Read the model definition and answer for the solid it produces. Units are mm, in the model's axes. A direction names the side the tool comes from. Coordinates: 2 decimals unless noted, no trailing zeros. Write each loop counter-clockwise with the first axis right and the second up, starting at its lowest first coordinate (ties: lowest second). Pieces come first, ordered by that corner, then holes. Notation, with made-up numbers: (-24.75, -30.75) -> (31.25, -30.75) arc R15 ccw to (31.25, -8.75) -> close; hole circle Ø2 at (-31, -37.75). An arc over 180 degrees is marked (long way). Return JSON: item names as keys, results as strings.
from build123d import *

# Parameters (mm, degrees)
SKETCH1_W           = 14.605
SKETCH1_H           = 46.482
SKETCH1_R           = 1.905
BOSS_EXTRUDE1_DEPTH = 44.45
SKETCH2_W           = 4.445
SKETCH2_H           = 33.02
CUT_EXTRUDE1_DEPTH  = 38.1
SKETCH3_W           = 42.545
SKETCH3_H           = 25.4
CUT_EXTRUDE2_DEPTH  = 12.065
CUT_EXTRUDE3_DEPTH  = 40.64
SKETCH5_W           = 25.4
SKETCH5_H           = 46.482
BOSS_EXTRUDE2_DEPTH = 3.81
FILLET1_R           = 2.54
FILLET2_R           = 1.016
CHAMFER1_SIZE       = 7.62
BOSS_EXTRUDE3_START = -7.62
BOSS_EXTRUDE3_DEPTH = 2.54
FILLET4_R           = 2.54


with BuildPart() as part:
    # Sketch1 → Boss-Extrude1 (new body)
    with BuildSketch(Plane.XY):
        with Locations((7.3025, 23.241)):
            Rectangle(SKETCH1_W, SKETCH1_H)
        with Locations((4.191, 42.291)):
            Circle(SKETCH1_R, mode=Mode.SUBTRACT)
        with Locations((4.191, 4.191)):
            Circle(SKETCH1_R, mode=Mode.SUBTRACT)
    extrude(amount=BOSS_EXTRUDE1_DEPTH)

    # Sketch2 → Cut-Extrude1 (cut)
    with BuildSketch(Plane.XY.offset(44.45)):
        with Locations((11.1125, 23.241)):
            Rectangle(SKETCH2_W, SKETCH2_H)
    extrude(amount=-CUT_EXTRUDE1_DEPTH, mode=Mode.SUBTRACT)

    # Sketch3 → Cut-Extrude2 (cut)
    with BuildSketch(Plane.ZY.offset(-13.335)):
        with Locations((21.2725, 23.241)):
            Rectangle(SKETCH3_W, SKETCH3_H)
    extrude(amount=CUT_EXTRUDE2_DEPTH, mode=Mode.SUBTRACT)

    # Sketch4 → Cut-Extrude3 (cut)
    with BuildSketch(Plane.XY.offset(44.45)):
        with BuildLine():
            Line((4.191, 38.1), (0, 38.1))
            Line((0, 38.1), (0, 46.482))
            Line((0, 46.482), (8.382, 46.482))
            Line((8.382, 46.482), (8.382, 42.291))
            ThreePointArc((8.382, 42.291), (7.15448452, 39.32751548), (4.191, 38.1))
        make_face()
        with BuildLine():
            Line((4.191, 8.382), (0, 8.382))
            Line((0, 8.382), (0, 0))
            Line((0, 0), (8.382, 0))
            Line((8.382, 0), (8.382, 4.191))
            ThreePointArc((8.382, 4.191), (7.15448452, 7.15448452), (4.191, 8.382))
        make_face()
    extrude(amount=-CUT_EXTRUDE3_DEPTH, mode=Mode.SUBTRACT)

    # Sketch5 → Boss-Extrude2 (add)
    with BuildSketch(Plane(origin=(0, 0, 0), x_dir=(-1, 0, 0), z_dir=(0, 0, -1))):
        with Locations((-27.305, 23.241)):
            Rectangle(SKETCH5_W, SKETCH5_H)
    extrude(amount=-BOSS_EXTRUDE2_DEPTH)

    # Fillet1
    fillet1_edges = [part.edges().sort_by_distance(p)[0] for p in [
        (8.382, 46.482, 24.13),
        (0, 38.1, 24.13),
        (0, 8.382, 24.13),
        (8.382, 0, 24.13),
        (0, 0, 1.905),
        (14.605, 0, 24.13),
        (14.605, 46.482, 24.13),
        (0, 46.482, 1.905),
        (40.005, 0, 1.905),
        (40.005, 46.482, 1.905),
    ]]
    fillet(fillet1_edges, radius=FILLET1_R)

    # Fillet2
    fillet2_edges = [part.edges().sort_by_distance(p)[0] for p in [
        (11.4935, 0, 44.45),
        (0, 23.241, 44.45),
        (11.4935, 46.482, 44.45),
        (8.382, 3.3655, 44.45),
        (14.605, 23.241, 44.45),
        (3.3655, 38.1, 44.45),
        (13.861051224, 45.738051224, 44.45),
        (13.861051224, 0.743948776, 44.45),
        (9.125948776, 0.743948776, 44.45),
        (0.743948776, 9.125948776, 44.45),
        (0.743948776, 37.356051224, 44.45),
        (9.125948776, 45.738051224, 44.45),
        (7.15448452, 39.32751548, 44.45),
        (8.382, 43.1165, 44.45),
        (7.15448452, 7.15448452, 44.45),
        (3.3655, 8.382, 44.45),
    ]]
    fillet(fillet2_edges, radius=FILLET2_R)

    # Chamfer1
    chamfer1_edges = [part.edges().sort_by_distance(p)[0] for p in [
        (1.27, 23.241, 42.545),
    ]]
    chamfer(chamfer1_edges, length=CHAMFER1_SIZE - 0.0001)  # a hair under: the kernel refuses the full size

    # Sketch6 → Boss-Extrude3 (add)
    with BuildSketch(Plane.XZ.offset(BOSS_EXTRUDE3_START)):
        Polygon((14.605, 22.86), (33.655, 3.81), (14.605, 3.81), align=None)
    boss_extrude3 = extrude(amount=-BOSS_EXTRUDE3_DEPTH)

    # Mirror1: Boss-Extrude3 across plane
    add(boss_extrude3.mirror(Plane(origin=(0, 23.241, 0), x_dir=(0, 0, 1), z_dir=(0, -1, 0))))

    # Fillet4
    fillet4_edges = [part.edges().sort_by_distance(p)[0] for p in [
        (14.605, 8.89, 22.86),
        (33.655, 8.89, 3.81),
        (14.605, 37.592, 22.86),
        (33.655, 37.592, 3.81),
    ]]
    fillet(fillet4_edges, radius=FILLET4_R)


solid = part.part
1. A tool of negligible diameter and unlimited length cuts with its end or side. For faces 5 (the face through (20, 36.322, 10)), 6 (the face through (8.382, 3, 24)), 7 (the face through (20, 38.862, 10)), 8 (the face through (1.27, 23, 17)), 9 (the face through (2, 42, 3.81)), from which of +Z, -Z, +X, -X, +Y, -Y can it reach the whole face along a straight path? Write none if from no direction.
Taken from the geometry:
{"face 5": "+Z, +X", "face 6": "+Z, -X, -Y", "face 7": "+Z, +X, +Y", "face 8": "-Z", "face 9": "+Z, -X, +Y"}
2. Flat-ended cylindrical pins translate along their axes: pin 1 Ø6 at (x, y) = (4.5, 14) entering from -Z; pin 2 Ø6 at (x, z) = (16.5, 8.5) entering from +Y; pin 3 Ø0.8 at (y, z) = (4, 25.5) entering from -X. Find the tip coordinate at first contact, or state that the pin passes through.
Taken from the geometry:
{"pin 1": "stops at z = 35.16", "pin 2": "stops at y = 46.04", "pin 3": "stops at x = 8.38"}
3. For a pull along X with two mould halves and no side action, classify faces 1 (the face through (9.11, 45.72, 23.34)), 2 (the face through (11, 38, 6.35)), 3 (the face through (5.133, 23.063, 38.788)), 4 (the face through (17, 46.482, 2)) as +X half, -X half, draft (parallel to the pull), parting line (faces both ways), or undercut.
Taken from the geometry:
{"face 1": "-X half", "face 2": "undercut", "face 3": "undercut", "face 4": "draft"}
4. The part is cut by section C-C (x = 18). Determine the outline of the cut face in (y, z) (3 decimals), then the cut area to 3 significant figures.
Taken from the geometry:
{"outline": "(0, 0) -> (46.482, 0) -> (46.482, 3.81) -> (38.862, 3.81) -> (38.862, 19.465) -> (36.322, 19.465) -> (36.322, 3.81) -> (10.16, 3.81) -> (10.16, 19.465) -> (7.62, 19.465) -> (7.62, 3.81) -> (0, 3.81) -> close", "area": "257 mm2"}
5. The part is cut by section B-B (z = 33.5). Determine the outline of the cut face in (x, y) (3 decimals).
Taken from the geometry:
{"outline": "(0, 10.922) arc R2.54 ccw to (2.54, 8.382) -> (4.191, 8.382) arc R4.191 cw to (8.382, 4.191) -> (8.382, 2.54) arc R2.54 ccw to (10.922, 0) -> (12.065, 0) arc R2.54 ccw to (14.605, 2.54) -> (14.605, 43.942) arc R2.54 ccw to (12.065, 46.482) -> (10.922, 46.482) arc R2.54 ccw to (8.382, 43.942) -> (8.382, 42.291) arc R4.191 cw to (4.191, 38.1) -> (2.54, 38.1) arc R2.54 ccw to (0, 35.56) -> close; hole (1.27, 10.541) -> (8.89, 10.541) -> (8.89, 6.731) -> (13.335, 6.731) -> (13.335, 39.751) -> (8.89, 39.751) -> (8.89, 35.941) -> (1.27, 35.941) -> close"}
6. Consider L1, parallel to X at y = 11, z = 30 (3 decimals); L2, parallel to Y at x = 23.5, z = 13; L3, parallel to Y at x = 4.5, z = 2.5. Determine where each line is inside the solid, lowest interval first.
Taken from the geometry:
{"L1": "x = 0 to 1.27, 13.335 to 14.605", "L2": "y = 7.62 to 10.16, 36.32 to 38.86", "L3": "y = 0 to 2.31, 6.07 to 10.54, 35.94 to 40.41, 44.17 to 46.48"}
